Verification items for the finished model (mm, model axes). Round coordinates to 2 decimals unless told otherwise and drop trailing zeros. Order: outer loops, then holes, each group sorted by start corner. A loop starts at its lowest first (then second) coordinate and runs counter-clockwise, first axis right, second up. Notation, with made-up numbers: (87, 61) -> (97, 61) arc R16 ccw to (97, 65) -> close; hole circle Ø11 at (37.5, -30.75). An arc over 180 degrees is marked (long way). Write item = value, one per line. Start each with the question number.
from build123d import *

# Parameters (mm, degrees)
SKETCH_1_W                = 200
SKETCH_1_H                = 270
EXTRUDE_1_DEPTH           = 16
HOLE_WIZARD_1_D           = 11
HOLE_WIZARD_1_CBORE_D     = 18
HOLE_WIZARD_1_CBORE_DEPTH = 11
CUT_EXTRUDE_1_DEPTH       = 169.763147636
SKETCH_5_W                = 150
SKETCH_5_H                = 180
CUT_EXTRUDE_2_DEPTH       = 169.763147636
FILLET_1_R                = 10
CHAMFER_1_SIZE            = 10
CHAMFER_2_SIZE            = 2


with BuildPart() as part:
    # 草图1 → 凸台-拉伸1 (new body)
    with BuildSketch(Plane.XY):
        Rectangle(SKETCH_1_W, SKETCH_1_H)
    extrude(amount=EXTRUDE_1_DEPTH)

    # 打孔尺寸(%根据)内六角圆柱头螺钉的类型1 (through all)
    with Locations(Plane(origin=(0, 0, 0), x_dir=(-1, 0, 0), z_dir=(0, 0, -1))):
        with Locations((-50, -116), (50, -116), (-50, 104), (50, 104)):
            CounterBoreHole(HOLE_WIZARD_1_D / 2, HOLE_WIZARD_1_CBORE_D / 2, HOLE_WIZARD_1_CBORE_DEPTH)

    # 草图4 → 切除-拉伸1 (cut, through all)
    with BuildSketch(Plane.XY.offset(16)):
        with BuildLine():
            Line((-88.3, 112.5), (-88.3, 117.5))
            ThreePointArc((-88.3, 117.5), (-85, 120.8), (-81.7, 117.5))
            Line((-81.7, 117.5), (-81.7, 112.5))
            ThreePointArc((-81.7, 112.5), (-85, 109.2), (-88.3, 112.5))
        make_face()
        with BuildLine():
            Line((81.7, 112.5), (81.7, 117.5))
            ThreePointArc((81.7, 117.5), (85, 120.8), (88.3, 117.5))
            Line((88.3, 117.5), (88.3, 112.5))
            ThreePointArc((88.3, 112.5), (85, 109.2), (81.7, 112.5))
        make_face()
        with BuildLine():
            Line((81.7, 72.5), (81.7, 77.5))
            ThreePointArc((81.7, 77.5), (85, 80.8), (88.3, 77.5))
            Line((88.3, 77.5), (88.3, 72.5))
            ThreePointArc((88.3, 72.5), (85, 69.2), (81.7, 72.5))
        make_face()
        with BuildLine():
            Line((-88.3, 72.5), (-88.3, 77.5))
            ThreePointArc((-88.3, 77.5), (-85, 80.8), (-81.7, 77.5))
            Line((-81.7, 77.5), (-81.7, 72.5))
            ThreePointArc((-81.7, 72.5), (-85, 69.2), (-88.3, 72.5))
        make_face()
        with BuildLine():
            Line((-88.3, -47.5), (-88.3, -42.5))
            ThreePointArc((-88.3, -42.5), (-85, -39.2), (-81.7, -42.5))
            Line((-81.7, -42.5), (-81.7, -47.5))
            ThreePointArc((-81.7, -47.5), (-85, -50.8), (-88.3, -47.5))
        make_face()
        with BuildLine():
            Line((-88.3, -87.5), (-88.3, -82.5))
            ThreePointArc((-88.3, -82.5), (-85, -79.2), (-81.7, -82.5))
            Line((-81.7, -82.5), (-81.7, -87.5))
            ThreePointArc((-81.7, -87.5), (-85, -90.8), (-88.3, -87.5))
        make_face()
        with BuildLine():
            Line((81.7, -47.5), (81.7, -42.5))
            ThreePointArc((81.7, -42.5), (85, -39.2), (88.3, -42.5))
            Line((88.3, -42.5), (88.3, -47.5))
            ThreePointArc((88.3, -47.5), (85, -50.8), (81.7, -47.5))
        make_face()
        with BuildLine():
            Line((81.7, -87.5), (81.7, -82.5))
            ThreePointArc((81.7, -82.5), (85, -79.2), (88.3, -82.5))
            Line((88.3, -82.5), (88.3, -87.5))
            ThreePointArc((88.3, -87.5), (85, -90.8), (81.7, -87.5))
        make_face()
    extrude(amount=-CUT_EXTRUDE_1_DEPTH, mode=Mode.SUBTRACT)

    # 草图5 → 切除-拉伸2 (cut, through all)
    with BuildSketch(Plane(origin=(0, 0, 0), x_dir=(-1, 0, 0), z_dir=(0, 0, -1))):
        Rectangle(SKETCH_5_W, SKETCH_5_H)
    extrude(amount=-CUT_EXTRUDE_2_DEPTH, mode=Mode.SUBTRACT)

    # 圆角1
    fillet_1_edges = [part.edges().sort_by_distance(p)[0] for p in [
        (75, -90, 8),
        (75, 90, 8),
        (-75, 90, 8),
        (-75, -90, 8),
    ]]
    fillet(fillet_1_edges, radius=FILLET_1_R)

    # 倒角1
    chamfer_1_edges = [part.edges().sort_by_distance(p)[0] for p in [
        (100, -135, 8),
        (-100, -135, 8),
        (-100, 135, 8),
        (100, 135, 8),
    ]]
    chamfer(chamfer_1_edges, length=CHAMFER_1_SIZE)

    # 倒角2
    chamfer_2_edges = [part.edges().sort_by_distance(p)[0] for p in [
        (0, 90, 0),
        (0, 90, 16),
        (-75, 0, 0),
        (-75, 0, 16),
        (75, 0, 0),
        (75, 0, 16),
        (0, -90, 0),
        (0, -90, 16),
        (-72.071067812, 87.071067812, 0),
        (-72.071067812, 87.071067812, 16),
        (72.071067812, 87.071067812, 0),
        (72.071067812, 87.071067812, 16),
        (-72.071067812, -87.071067812, 0),
        (-72.071067812, -87.071067812, 16),
        (72.071067812, -87.071067812, 0),
        (72.071067812, -87.071067812, 16),
        (100, 0, 0),
        (100, 0, 16),
        (0, -135, 0),
        (-100, 0, 0),
        (0, 135, 0),
        (-95, -130, 0),
        (-95, 130, 0),
        (95, 130, 0),
        (95, -130, 0),
        (0, -135, 16),
        (0, 135, 16),
        (-100, 0, 16),
        (-95, -130, 16),
        (-95, 130, 16),
        (95, 130, 16),
        (95, -130, 16),
    ]]
    chamfer(chamfer_2_edges, length=CHAMFER_2_SIZE)


solid = part.part
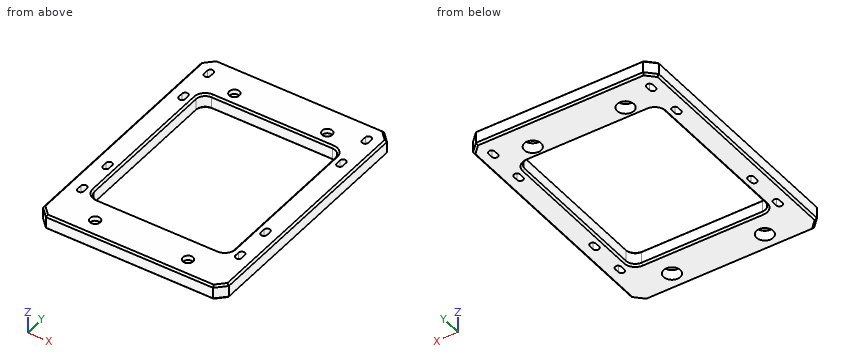
(1) Cross-section at A-A (y = 55.5). Enter the section's corners in (x, z).
(2) Cross-section at D-D (y = -116). Enter the section's corners in (x, z).
(3) Scan lines: line 1 along Y through (x, z) = (50, 12.5); line 2 along Y through (x, z) = (-50, 7); line 3 along Y through (x, z) = (83.5, 4). Record each from-to range of solid material in increasing order. Write a range as from..to.
(4) Depth check by flat-ended pin: pin 1 (17.5 mm diameter, centred on x = 50, y = 104, fed in from -Z); pin 2 (10 mm diameter, centred on x = -50, y = 104, fed in from +Z). Enter the tip coordinate at first touch or a pass-through.
(5) Cross-section at C-C (x = -50). Give the number of separate pieces and of enclosed holes in the cut face, and give its area (3 significant figures).
(6) Cross-section at B-B (x = 85). Enter the section's corners in (y, z).
Outcome:
q1.outline = (-100, 2) -> (-98, 0) -> (-77, 0) -> (-75, 2) -> (-75, 14) -> (-77, 16) -> (-98, 16) -> (-100, 14) -> close; (75, 2) -> (77, 0) -> (98, 0) -> (100, 2) -> (100, 14) -> (98, 16) -> (77, 16) -> (75, 14) -> close
q2.outline = (-100, 2) -> (-98, 0) -> (-59, 0) -> (-59, 11) -> (-55.5, 11) -> (-55.5, 16) -> (-98, 16) -> (-100, 14) -> close; (-44.5, 11) -> (-41, 11) -> (-41, 0) -> (41, 0) -> (41, 11) -> (44.5, 11) -> (44.5, 16) -> (-44.5, 16) -> close; (55.5, 11) -> (59, 11) -> (59, 0) -> (98, 0) -> (100, 2) -> (100, 14) -> (98, 16) -> (55.5, 16) -> close
q3.line_1 = -135..-121.5, -110.5..-90, 90..98.5, 109.5..135
q3.line_2 = -135..-125, -107..-90, 90..95, 113..135
q3.line_3 = -135..-90.44, -79.56..-50.44, -39.56..69.56, 80.44..109.56, 120.44..135
q4.pin_1 = 11
q4.pin_2 = through
q5.separate_pieces = 4
q5.enclosed_holes = 0
q5.area = 918 mm^2
q6.outline = (-135, 2) -> (-133, 0) -> (-90.8, 0) -> (-90.8, 16) -> (-133, 16) -> (-135, 14) -> close; (-79.2, 0) -> (-50.8, 0) -> (-50.8, 16) -> (-79.2, 16) -> close; (-39.2, 0) -> (69.2, 0) -> (69.2, 16) -> (-39.2, 16) -> close; (80.8, 0) -> (109.2, 0) -> (109.2, 16) -> (80.8, 16) -> close; (120.8, 0) -> (133, 0) -> (135, 2) -> (135, 14) -> (133, 16) -> (120.8, 16) -> close
